Input: dimensioned drawing with shaded views. Units: mm. Origin: part minimum x, y, z. Round coordinates to 2 decimals unless told otherwise and drop trailing zeros. Order: outer loops, then holes, each group sorted by start corner. A loop starts at its lowest first (then second) coordinate and runs counter-clockwise, first axis right, second up. Notation, with made-up numbers: (48, 65) - (94, 65) arc R20 ccw to (94, 70) - close; hole circle Ø3 at (66, 32.25). An arc over 180 degrees is marked (long way). Put each result on its own line as item: value. Start each with the question number.
(1) Pull-direction query (Z, two-part tool) for the marked faces 1, 2 and 3; classes: released by +Z, released by -Z, zero draft, split by the parting line, or undercut.
(2) Section D-D (z = 19.25). Output: boundary loops of the cut face in (x, y), and give its area (3 significant figures).
(3) Material intervals for L1, parallel to Z at x = 32.5, y = 2.05 (1 decimal); L2, parallel to Z at x = 31.75, y = 1.7; L3, parallel to X at y = 1.5, z = 32.5, sorted ascending. Write a range as [from, to].
(4) Section B-B (x = 20.5). Output: boundary loops of the cut face in (y, z) (1 decimal).
(5) Pin query (flat end, axial travel): P1, Ø2.5, axis at x = 10.1, z = 19.25, coming from the +Y side; P2, Ø2, axis at x = 31.5, y = 1.5, coming from the +Z side; P3, Ø1, axis at x = 42.5, y = 2.5, coming from the +Z side; P4, Ø1, axis at x = 27.5, y = 4, coming from the +Z side. Return the tip coordinate at first contact, or that it passes through.
(6) Section A-A (z = 31.75). Output: boundary loops of the cut face in (x, y).
(7) Section C-C (x = 31.75). Output: boundary loops of the cut face in (y, z).
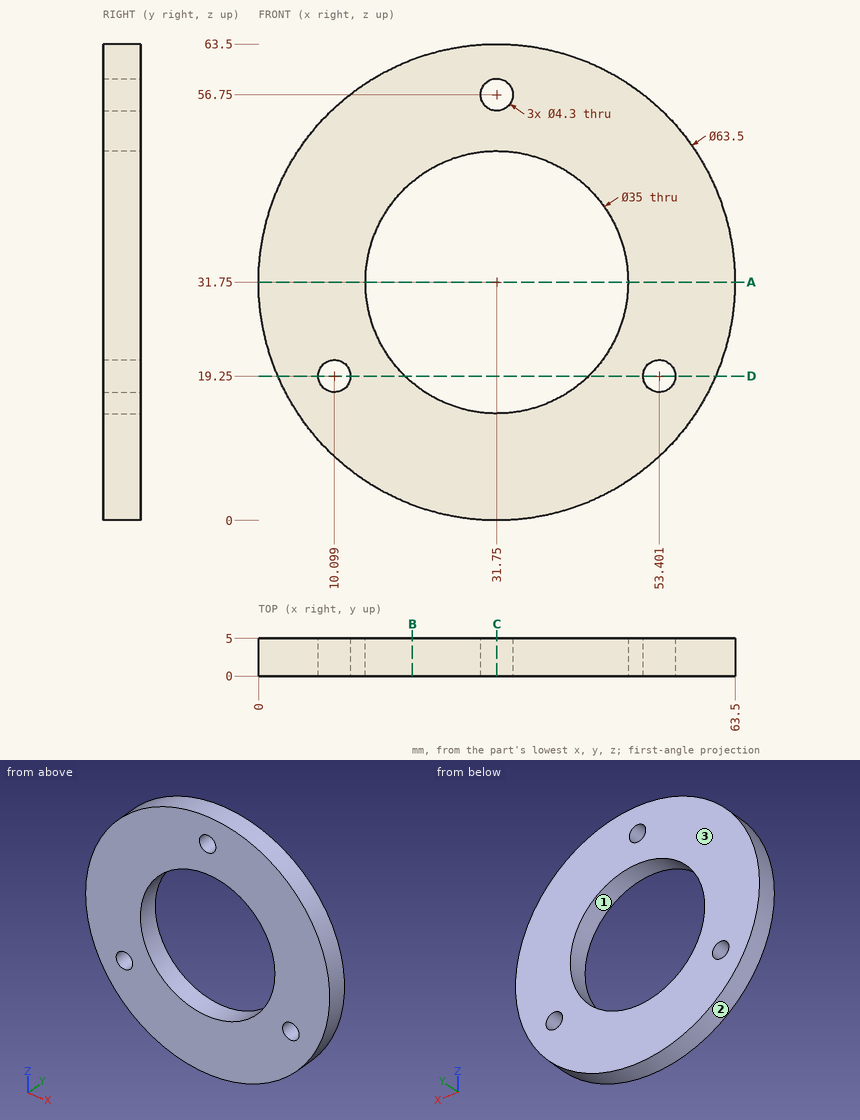
Checks:
1. face 1: undercut
1. face 2: split by the parting line
1. face 3: zero draft
2. outline: (2.56, 0) - (7.95, 0) - (7.95, 5) - (2.56, 5) - close; (12.25, 0) - (19.5, 0) - (19.5, 5) - (12.25, 5) - close; (44, 0) - (51.25, 0) - (51.25, 5) - (44, 5) - close; (55.55, 0) - (60.94, 0) - (60.94, 5) - (55.55, 5) - close
2. area: 126 mm²
3. L1: z = [0, 14.3], [49.2, 54.7], [58.8, 63.5]
3. L2: z = [0, 14.25], [49.25, 54.6], [58.9, 63.5]
3. L3: x = [0.01, 14.27], [49.23, 63.49]
4. outline: (0, 2.1) - (5, 2.1) - (5, 18.3) - (0, 18.3) - close; (0, 45.2) - (5, 45.2) - (5, 61.4) - (0, 61.4) - close
5. P1: passes through
5. P2: stops at z = 63.5
5. P3: stops at z = 61.8
5. P4: stops at z = 63.28
6. outline: (0, 0) - (14.25, 0) - (14.25, 5) - (0, 5) - close; (49.25, 0) - (63.5, 0) - (63.5, 5) - (49.25, 5) - close
7. outline: (0, 0) - (5, 0) - (5, 14.25) - (0, 14.25) - close; (0, 49.25) - (5, 49.25) - (5, 54.6) - (0, 54.6) - close; (0, 58.9) - (5, 58.9) - (5, 63.5) - (0, 63.5) - close
